Check sheet for the modelled part. Datum: model origin and axes. Units: mm. A direction names the side the tool comes from. Coordinates: 2 decimals unless noted, no trailing zeros. Loops run counter-clockwise (first coordinate to the right, second up) from the corner with the lowest first, then second, coordinate; pieces in that order, holes last. Notation, with made-up numbers: (36.25, 36) -> (87.25, 36) arc R18 cw to (87.25, 53) -> close; hole circle Ø7 at (-34.75, -5.75). An arc over 180 degrees is marked (long way). Use one line per item in the form item = value.
Autodesk Inventor part; units mm, degrees
ref_plane "YZ Plane" through (0, 0, 0) normal (1, 0, 0) x (0, 1, 0)
ref_plane "XZ Plane" through (0, 0, 0) normal (0, 1, 0) x (-1, 0, 0)
ref_plane "XY Plane" through (0, 0, 0) normal (0, 0, 1) x (1, 0, 0)
sketch "草图1" plane through (42.95, 80.9918, 0) normal (0, 0, -1) x (-1, 0, 0)
  line L0 (-94.1, 15) -> (0, 15)
  line L1 (0, 15) -> (0, -1)
  line L2 (0, -1) -> (-94.1, -1)
  line L3 (-94.1, -1) -> (-94.1, 15)
  line L4 (0, 0) -> (0, 14)
  line L5 (-94.1, 14) -> (-94.1, 0)
  line L6 (0, 14) -> (-94.1, 14)
  line L7 (-94.1, 0) -> (0, 0)
  line L8 (-94.1, 7) -> (0, 7)
  line L9 (-39.1, -4.5) -> (-94.1, -4.5)
  line L10 (-94.1, -4.5) -> (-94.1, 18.5)
  line L11 (-94.1, 18.5) -> (-39.1, 18.5)
  line L12 (-39.1, 18.5) -> (-39.1, -4.5)
  line L13 (-39.1, -4.5) -> (-94.1, 18.5) construction
  line L14 (-94.1, -4.5) -> (-39.1, 18.5) construction
  point P0 (42.95, -80.9918)
  point P1 (-66.6, 7)
  point P2 (-39.1, -1)
  point P3 (-39.1, 15)
  dimension "d0" = 1
  dimension "d1" = 1
  dimension "d2" = 23
  dimension "d3" = 55
extrude "拉伸1" add sketch "草图1" along normal blind 1
sketch "草图2" plane through (42.95, 80.9918, -1) normal (0, 0, -1) x (-1, 0, 0)
  line L0 (-74.55, 0) -> (-74.55, -4.5)
  line L1 (-39.1, 18.5) -> (-94.1, 18.5)
  line L2 (-94.1, -4.5) -> (-39.1, -4.5)
  line L3 (-39.1, -4.5) -> (-39.1, 18.5)
  line L4 (-39.1, 18.5) -> (-94.1, 18.5)
  line L5 (-94.1, 18.5) -> (-94.1, -4.5)
  line L6 (-96.1, -6.5) -> (-37.1, -6.5)
  line L7 (-37.1, -6.5) -> (-37.1, 20.5)
  line L8 (-37.1, 20.5) -> (-96.1, 20.5)
  line L9 (-96.1, 20.5) -> (-96.1, -6.5)
  point P0 (42.95, -80.9918)
  dimension "d6" = 2
extrude "拉伸2" add sketch "草图2" against normal up to surface (1 mm away) contours L3 L2 L5 L1 | L9 L8 L7 L6
extrude "拉伸3" add sketch "草图2" along normal blind 15
fillet "圆角1" radius 2 1 edges at (80.05, 87.9918, -1)
sketch "草图3" plane through (42.95, 80.9918, 0) normal (0, 0, 1) x (1, 0, 0)
  point P0 (-42.95, -80.9918)
fillet "圆角2" radius 3 4 edges at (80.05, 74.4918, -8) (80.05, 101.4918, -8) (139.05, 74.4918, -8) (139.05, 101.4918, -8)
sketch "草图4" plane through (42.95, 79.9918, -1) normal (0, -1, 0) x (1, 0, 0)
  line L0 (0, 1) -> (0, 0)
  line L1 (37.1, 1) -> (37.1, -15)
  line L2 (0, 0) -> (37.1, 0)
  line L3 (37.1, 0) -> (37.1, -9.5558)
  line L4 (37.1, -9.5558) -> (0, -9.5558)
  line L5 (0, -9.5558) -> (0, 0)
  point P0 (-42.95, 1)
  point P1 (37.1, 0)
extrude "拉伸4" add sketch "草图4" against normal up to surface (16 mm away)
fillet "圆角3" radius 5.5 1 edges at (80.05, 87.9918, -10.5558)
sketch "草图5" plane through (42.95, 79.9918, 0) normal (0, -1, 0) x (1, 0, 0)
  line L0 (0, 0) -> (37.1, 0)
  line L1 (0, 0) -> (37.1, 0)
  line L2 (37.1, 0) -> (37.1, -3)
  line L3 (37.1, -3) -> (0, -3)
  line L4 (0, -3) -> (0, 0)
  line L5 (37.1, 0) -> (37.1, -16)
  line L6 (0, -3) -> (37.2428, -3)
  line L7 (37.2428, -3) -> (37.2428, -6.4975)
  line L8 (37.2428, -6.4975) -> (0, -6.4975)
  line L9 (0, -6.4975) -> (0, -3)
  line L10 (0, 0) -> (0, -10.5558)
  line L11 (0, -4) -> (23.3302, -6.4975)
  point P0 (-42.95, 0)
  point P1 (0, -4)
  point P2 (37.1, -7.9715)
  point P3 (37.1, -3)
  point P4 (37.1, -6.4975)
  dimension "d16" = 3
  dimension "d20" = 1
extrude "拉伸5" cut sketch "草图5" against normal blind 61.75 contours L3 L5 L8 L11 L9
fillet "圆角4" radius 1 3 edges at (80.05, 87.9918, -3) (42.95, 87.9918, -4) (42.95, 87.9918, -3)
sketch "草图6" plane through (42.95, 80.9918, 0) normal (0, 0, 1) x (1, 0, 0)
  circle A0 centre (44.1719, 16.2818) radius 2
  point P0 (-42.95, -80.9918)
  dimension "d22" = 4
extrude "拉伸6" cut sketch "草图6" against normal blind 61.75
properties part number "obj_1_电池盒.STEP_3D 打印"
(1) Scan lines: line 1 along X through (y, z) = (91, -10.25); line 2 along Y through (x, z) = (104, -4); line 3 along X through (y, z) = (98, -8). Record each from-to range of solid material in increasing order.
Established:
line_1 = 42.95 to 82.05, 137.05 to 139.05
line_2 = 74.49 to 76.49, 99.49 to 101.49
line_3 = 80.05 to 82.05, 137.05 to 139.05
(2) Section check C-C, the plane y = 91.5. Record the boundary of the cut face in (x, z), plus the area to 3 significant figures.
Established:
outline = (42.95, -10.56) -> (74.55, -10.56) arc R5.5 cw to (80.05, -16) -> (82.05, -16) -> (82.05, -1) -> (137.05, -1) -> (137.05, -16) -> (139.05, -16) -> (139.05, 0) -> (42.95, 0) -> (42.95, -2) arc R1 ccw to (43.95, -3) -> (79.05, -3) arc R1 cw to (80.05, -4) -> (80.05, -6.5) -> (66.28, -6.5) -> (44.06, -4.12) arc R1 ccw to (42.95, -5.11) -> close
area = 416 mm²
(3) Section check B-B, the plane x = 49.5. Record the boundary of the cut face in (y, z).
Established:
outline = (79.99, -10.56) -> (95.99, -10.56) -> (95.99, -4.7) -> (79.99, -4.7) -> close; (79.99, -3) -> (95.99, -3) -> (95.99, 0) -> (79.99, 0) -> close
(4) Go/stop test with flat-tipped pins: P1, Ø9.5, axis at x = 59, z = -13, coming from the +Y side; P2, Ø3.5, axis at x = 87.12, y = 97.27, coming from the +Z side; P3, Ø13, axis at x = 61, y = 90, coming from the -Z side; P4, Ø11.5, axis at x = 122.5, y = 87, coming from the -Z side. Record where each tip stops, or that it passes through.
Established:
P1 = 95.99
P2 = through
P3 = -10.56
P4 = -1
(5) Section check D-D, the plane x = 105. Record the boundary of the cut face in (y, z).
Established:
outline = (74.49, -16) -> (76.49, -16) -> (76.49, -1) -> (99.49, -1) -> (99.49, -16) -> (101.49, -16) -> (101.49, 0) -> (74.49, 0) -> close
(6) Tool access check on faces 4 (the flat face through (110, 88, -1)), 5 (the flat face through (55.01, 87.88, -5.29)), 6 (the flat face through (61, 95.992, -2)), 7 (the flat face through (59, 88, -10.556)), 8 (the flat face through (61, 79.992, -9)). Record the directions out of +Z, -Z, +X, -X, +Y, -Y that give a thin tool (end or side, any length) a straight path to the whole face; none if there is none.
Established:
face_4 = -Z
face_5 = +Y, -Y
face_6 = +Z, -Z, -X, +Y
face_7 = -Z, -X, +Y, -Y
face_8 = +Z, -Z, -X, -Y
(7) Mould release check, pull along Y, two halves, no side actions. Record for faces 1 (the cylindrical face through (138.195, 100.59, -7.888)), 2 (the flat face through (109, 99.492, -8)), 3 (the cylindrical face through (138.2, 75.4, -8.1)): +Y half, -Y half, draft (parallel to the pull), parting line (faces both ways), or undercut.
Established:
face_1 = +Y half
face_2 = undercut
face_3 = -Y half
(8) Section check A-A, the plane z = -7.5. Record the boundary of the cut face in (x, y).
Established:
outline = (42.95, 79.99) -> (80.05, 79.99) -> (80.05, 77.49) arc R3 ccw to (83.05, 74.49) -> (136.05, 74.49) arc R3 ccw to (139.05, 77.49) -> (139.05, 98.49) arc R3 ccw to (136.05, 101.49) -> (83.05, 101.49) arc R3 ccw to (80.05, 98.49) -> (80.05, 95.99) -> (42.95, 95.99) -> close; hole (82.05, 76.49) -> (137.05, 76.49) -> (137.05, 99.49) -> (82.05, 99.49) -> close
